The model under review builds one solid part; all positions refer to its coordinate system, in mm. A direction names the side the tool comes from. Round coordinates to 2 decimals unless told otherwise and drop trailing zeros. Order: outer loops, then holes, each group sorted by start corner. A loop starts at its lowest first (then second) coordinate and runs counter-clockwise, first axis right, second up. Notation, with made-up numbers: M 32.5,50 L 38.5,50 A23 cw 38.5,81 Z; hole C -14,34 d10. An arc over 180 degrees is marked long. Answer as a JSON object with one key per item and string values. Group by question number.
1) To check wall thickness, follow line 1 (Z direction, x = 43.5, y = 97.5); line 2 (X direction, y = 87, z = 185); line 3 (Y direction, x = 193, z = 100). State the ranges of each line that lie inside material, in increasing order.
2) For faces 1 (the flat face through (290, 110, 179)), 2 (the flat face through (280, 75, 95)), 3 (the flat face through (20, 93, 179)), 4 (the flat face through (10, 75, 164)), list the 3-axis set-ups (+Z, -Z, +X, -X, +Y, -Y) from which the entire face can be reached by the end or side of a thin tool; tool diameter is ignored.
3) Consider section A-A, the plane z = 205.5. Write out the cut boundary in (x, y).
4) Consider section D-D, the plane z = 94.5. Write out the cut boundary in (x, y), then the cut area to 3 significant figures.
5) Consider section B-B, the plane x = 208. Write out the cut boundary in (y, z).
6) The part is to be moulded in two halves that separate along Y. For faces 5 (the flat face through (280, 92, 179)), 6 (the flat face through (148, 115, 179)), 7 (the flat face through (15, 80, 164)), 8 (the flat face through (290, 75, 164)), say which applies: +Y half, -Y half, draft (parallel to the pull), parting line (faces both ways), or undercut.
7) Insertion check: pin 1 Ø3 at (x, y) = (16, 75) entering from -Z; pin 2 Ø7.5 at (y, z) = (91.5, 184) entering from -X; pin 3 Ø11 at (x, z) = (13.5, 168.5) entering from -Y; pin 4 Ø5 at (y, z) = (77, 200) entering from +X. Each pin has a flat end and moves straight along its axis. Give the tip position at first contact, or say it passes through.
8) Consider section C-C, the plane y = 91.5. Write out the cut boundary in (x, z), then the cut area to 3 significant figures.
Autodesk Inventor part; units mm, degrees
ref_plane "YZ Plane" through (0, 0, 0) normal (1, 0, 0) x (0, 1, 0)
ref_plane "XZ Plane" through (0, 0, 0) normal (0, 1, 0) x (-1, 0, 0)
ref_plane "XY Plane" through (0, 0, 0) normal (0, 0, 1) x (1, 0, 0)
sketch "스케치1" plane through (0, 0, 0) normal (0, 0, 1) x (1, 0, 0)
  line L0 (0, 0) -> (300, 0)
  line L1 (300, 0) -> (300, 70)
  line L2 (300, 70) -> (280, 70)
  line L3 (280, 70) -> (280, 105)
  line L4 (20, 105) -> (20, 70)
  line L5 (20, 70) -> (0, 70)
  line L6 (0, 70) -> (0, 0)
  line L7 (20, 105) -> (10, 105)
  line L8 (10, 105) -> (10, 115)
  line L9 (10, 115) -> (290, 115)
  line L10 (290, 115) -> (290, 105)
  line L11 (290, 105) -> (280, 105)
  line L12 (20, 70) -> (280, 70)
  line L13 (10, 70) -> (10, 80)
  line L14 (10, 80) -> (20, 80)
  line L15 (150, 115) -> (150, 100)
  line L16 (290, 70) -> (290, 80)
  line L17 (290, 80) -> (280, 80)
  point P0 (150, 0)
  dimension "d0" = 300
  dimension "d1" = 70
  dimension "d2" = 35
  dimension "d3" = 20
  dimension "d4" = 10
  dimension "d5" = 10
  dimension "d10" = 10
extrude "돌출1" add sketch "스케치1" along normal blind 250
extrude "돌출2" cut sketch "스케치1" along normal blind 110 contours L4 L7 L8 L9 L10 L11 L3 L12
extrude "돌출3" cut sketch "스케치1" along normal blind 80 contours L13 L14 L4 L5 | L2 L3 L17 L16
properties part number "DummyModule"
Results list:
{
 "1": {"line 1": "110 to 250", "line 2": "20 to 280", "line 3": "0 to 70"},
 "2": {"face 1": "+Z, -Z, +X, +Y", "face 2": "-Z, +Y", "face 3": "+Z, -Z, -X", "face 4": "+Z, -Z, -X, +Y"},
 "3": {"outline": "M 0,0 L 300,0 L 300,70 L 290,70 L 290,80 L 280,80 L 280,105 L 290,105 L 290,115 L 10,115 L 10,105 L 20,105 L 20,80 L 10,80 L 10,70 L 0,70 Z"},
 "4": {"outline": "M 0,0 L 300,0 L 300,70 L 290,70 L 290,80 L 280,80 L 280,70 L 20,70 L 20,80 L 10,80 L 10,70 L 0,70 Z", "area": "21,200 mm^2"},
 "5": {"outline": "M 0,0 L 70,0 L 70,110 L 115,110 L 115,250 L 0,250 Z"},
 "6": {"face 5": "undercut", "face 6": "+Y half", "face 7": "undercut", "face 8": "draft"},
 "7": {"pin 1": "z = 80", "pin 2": "x = 20", "pin 3": "y = 0", "pin 4": "x = 290"},
 "8": {"outline": "M 20,110 L 280,110 L 280,250 L 20,250 Z", "area": "36,400 mm^2"}
}
